CAD build for the part. Positions are in the model's coordinates, mm. A direction names the side the tool comes from. Give positions to 0.01 mm unless a question says otherwise; leave off trailing zeros. Write each loop counter-clockwise with the first axis right and the second up, starting at its lowest first coordinate (ties: lowest second). Pieces come first, ordered by that corner, then holes. Notation, with made-up numbers: (11.5, 55) -> (31.5, 55) arc R18 cw to (31.5, 74) -> close; hole circle Ø1 at (15.25, 41). An arc over 180 degrees is marked (long way). Answer as a JSON object with one key per item and string values.
```python
from build123d import *

# Parameters (mm, degrees)
SKETCH1_R                = 6.35
SKETCH1_R_2              = 3.175
BOSS_EXTRUDE1_DEPTH      = 17.78
BOSS_EXTRUDE2_DEPTH      = 17.78
BOSS_EXTRUDE3_DEPTH      = 12.7
BOSS_EXTRUDE3_DEPTH_BACK = 30.48
FILLET1_R                = 10


with BuildPart() as part:
    # Sketch1 → Boss-Extrude1 (new body)
    with BuildSketch(Plane.XY):
        with Locations((-12.7, 137.7)):
            Circle(SKETCH1_R)
        with Locations((-12.7, 137.7)):
            Circle(SKETCH1_R_2, mode=Mode.SUBTRACT)
    extrude(amount=BOSS_EXTRUDE1_DEPTH)

    # Sketch2 → Boss-Extrude2 (add)
    with BuildSketch(Plane.XY.offset(17.78)):
        with BuildLine():
            Line((-12.7, 131.35), (-28.041116719, 131.35))
            Line((-28.041116719, 131.35), (-28.041116719, 144.05))
            Line((-28.041116719, 144.05), (-12.7, 144.05))
            ThreePointArc((-12.7, 144.05), (-19.05, 137.7), (-12.7, 131.35))
        make_face()
    extrude(amount=-BOSS_EXTRUDE2_DEPTH)

    # Sketch3 → Boss-Extrude3 (add, two sides)
    with BuildSketch(Plane.XY.offset(17.78)) as boss_extrude3_sk:
        with BuildLine():
            Line((-28.041116719, 131.35), (-28.041116719, 118.65))
            Line((-28.041116719, 118.65), (-31.216116719, 118.65))
            ThreePointArc((-31.216116719, 118.65), (-35.746712734, 150.055233925), (-13.026751575, 172.205140992))
            Line((-13.026751575, 172.205140992), (-10.387770933, 170.439806414))
            Line((-10.387770933, 170.439806414), (-25.897039285, 147.25515947))
            ThreePointArc((-25.897039285, 147.25515947), (-27.493281477, 143.883657427), (-28.041116719, 140.193821156))
            Line((-28.041116719, 140.193821156), (-28.041116719, 131.35))
        make_face()
    extrude(amount=BOSS_EXTRUDE3_DEPTH)
    extrude(boss_extrude3_sk.sketch, amount=-BOSS_EXTRUDE3_DEPTH_BACK)

    # Fillet1
    fillet1_edges = [part.edges().sort_by_distance(p)[0] for p in [
        (-28.041116719, 131.35, 8.89),
    ]]
    fillet(fillet1_edges, radius=FILLET1_R)


solid = part.part
```
1) Slice it at D-D (z = 27). List the corners of the cut face in (x, y).
Model answer:
{"outline": "(-31.22, 118.65) -> (-28.04, 118.65) -> (-28.04, 140.19) arc R12.7 cw to (-25.9, 147.26) -> (-10.39, 170.44) -> (-13.03, 172.21) arc R34.98 ccw to start"}
2) Slice it at B-B (y = 137.7). List the corners of the cut face in (x, z) (3 decimals).
Model answer:
{"outline": "(-37.588, -12.7) -> (-28.041, -12.7) -> (-28.041, 0) -> (-15.875, 0) -> (-15.875, 17.78) -> (-28.041, 17.78) -> (-28.041, 30.48) -> (-37.588, 30.48) -> close; (-9.525, 0) -> (-6.35, 0) -> (-6.35, 17.78) -> (-9.525, 17.78) -> close"}
3) Pin check, flat tips, straight feed: pin 1 (6.5 mm diameter, centred on x = -17, y = 135.5, fed in from +Z); pin 2 (12 mm diameter, centred on x = -19.5, z = 7.5, fed in from +Y); pin 3 (10 mm diameter, centred on y = 125, z = 12, fed in from +X). Stop position of each tip, or through.
Model answer:
{"pin 1": "stops at z = 17.78", "pin 2": "stops at y = 172.05", "pin 3": "stops at x = -23.06"}
4) Mould opens along X. For faces 1 (the cylindrical face through (-13.11, 140.85, 8.77)), 2 (the flat face through (-20, 138, 0)), 3 (the cylindrical face through (-6.35, 137.56, 8.77)) say: released by +X, released by -X, zero draft, split by the parting line, or undercut.
Model answer:
{"face 1": "undercut", "face 2": "zero draft", "face 3": "released by +X"}
5) 3-axis set-ups, long thin cutter, end or side, ignore diameter. For faces 4 (the flat face through (-15, 131.35, 9)), 5 (the flat face through (-18.034, 159.01, 9.192)), 6 (the flat face through (-28.041, 120, 9)): which of +Z, -Z, +X, -X, +Y, -Y reach the whole face in a straight line?
Model answer:
{"face 4": "+Z, -Z, +X, -Y", "face 5": "+Z, -Z, +X", "face 6": "+X, -Y"}
6) Slice it at A-A (z = 11). List the corners of the cut face in (x, y) (3 decimals).
Model answer:
{"outline": "(-31.216, 118.65) -> (-28.041, 118.65) -> (-28.041, 121.35) arc R10 cw to (-18.041, 131.35) -> (-12.7, 131.35) arc R6.35 ccw to (-12.7, 144.05) -> (-27.442, 144.05) arc R12.7 cw to (-25.897, 147.255) -> (-10.388, 170.44) -> (-13.027, 172.205) arc R34.984 ccw to start; hole circle Ø6.35 at (-12.7, 137.7)"}
7) Wall check: probe 1 along Y at (x, z) = (-12.7, 4.5) (3 decimals); probe 2 along X at (y, z) = (135.5, 14); probe 3 along Y at (x, z) = (-25, 16.5). Give the ranges that are in metal, low to high.
Model answer:
{"probe 1": "y = 131.35 to 134.525, 140.875 to 144.05, 166.983 to 171.987", "probe 2": "x = -37.45 to -14.99, -10.41 to -6.74", "probe 3": "y = 128.53 to 144.05, 148.6 to 165.69"}
8) Slice it at C-C (x = -21). List the corners of the cut face in (y, z).
Model answer:
{"outline": "(130.9, 0) -> (144.05, 0) -> (144.05, 17.78) -> (130.9, 17.78) -> close; (154.58, -12.7) -> (168.57, -12.7) -> (168.57, 30.48) -> (154.58, 30.48) -> close"}
